Could you check a few things on this drawing? It's one solid part, dimensions in mm from its lowest x, y, z. Round coordinates to 2 decimals unless told otherwise and drop trailing zeros. Write each loop counter-clockwise with the first axis right and the second up, starting at its lowest first coordinate (ties: lowest second). Pieces come first, ordered by that corner, then holes. Notation, with made-up numbers: (63, -30.75) -> (113, -30.75) arc R16 cw to (113, -20.75) -> close; hole circle Ø3 at (51, -14). An arc over 180 degrees is marked (long way). Return JSON: item names as keys, results as strings.
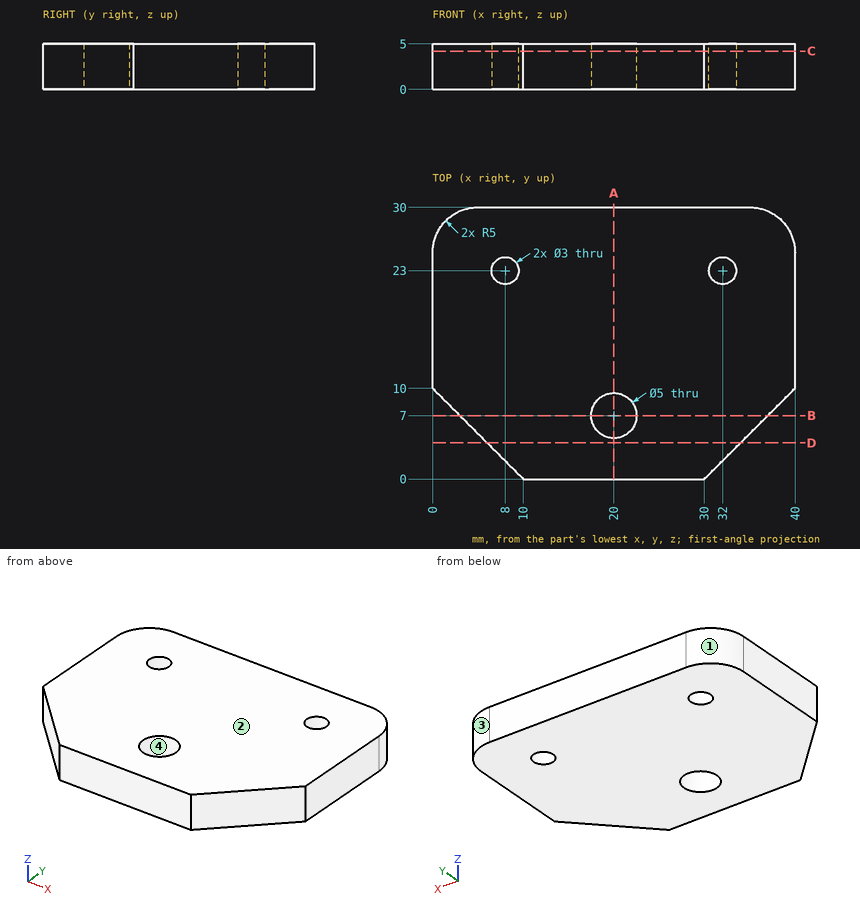
1) If I drill on probe 1 along Y at (x, z) = (20, 2.6); probe 2 along X at (y, z) = (21.75, 2.1); probe 3 along X at (y, z) = (7, 1.55), over which ranges is the centre line in solid material (lowest first)? Write a range as [from, to].
Return value:
{"probe 1": "[0, 4.5], [9.5, 30]", "probe 2": "[0, 7.17], [8.83, 31.17], [32.83, 40]", "probe 3": "[3, 17.5], [22.5, 37]"}
2) I want a section at B-B, the plane y = 7. Please give me the cut outline in (x, z).
Return value:
{"outline": "(3, 0) -> (17.5, 0) -> (17.5, 5) -> (3, 5) -> close; (22.5, 0) -> (37, 0) -> (37, 5) -> (22.5, 5) -> close"}
3) Thinking about a two-plate mould opening in X: for the marked faces 1, 2, 3 and 4, which applies, pulls with the +X half, pulls with the -X half, needs draft (parallel to the pull), parting line crosses it, or undercut?
Return value:
{"face 1": "pulls with the -X half", "face 2": "needs draft", "face 3": "pulls with the +X half", "face 4": "undercut"}
4) I want a section at D-D, the plane y = 4. Please give me the cut outline in (x, z), and give its area (3 significant figures).
Return value:
{"outline": "(6, 0) -> (34, 0) -> (34, 5) -> (6, 5) -> close", "area": "140 mm²"}
5) I want a section at C-C, the plane z = 4.2. Please give me the cut outline in (x, y), and give its area (3 significant figures).
Return value:
{"outline": "(0, 10) -> (10, 0) -> (30, 0) -> (40, 10) -> (40, 25) arc R5 ccw to (35, 30) -> (5, 30) arc R5 ccw to (0, 25) -> close; hole circle Ø3 at (8, 23); hole circle Ø5 at (20, 7); hole circle Ø3 at (32, 23)", "area": "1,060 mm²"}
6) Will these pins go through, and if not, where does the flat tip stop? pin 1 Ø4.5 at (x, y) = (20, 7) entering from +Z; pin 2 Ø3 at (x, y) = (10.5, 10.5) entering from -Z.
Return value:
{"pin 1": "through", "pin 2": "z = 0"}
7) I want a section at A-A, the plane x = 20. Please give me the cut outline in (y, z).
Return value:
{"outline": "(0, 0) -> (4.5, 0) -> (4.5, 5) -> (0, 5) -> close; (9.5, 0) -> (30, 0) -> (30, 5) -> (9.5, 5) -> close"}
